Check sheet for the modelled part. Datum: model origin and axes. Units: mm. A direction names the side the tool comes from. Give positions to 0.01 mm unless a question says otherwise; leave off trailing zeros. Loops run counter-clockwise (first coordinate to the right, second up) from the corner with the lowest first, then second, coordinate; pieces in that order, holes last. Notation, with made-up numbers: (5, 5) - (33, 5) arc R4 cw to (33, 10) - close; hole circle Ø11 at (52.5, 16). An arc over 180 degrees is marked (long way). Answer in a Markdown table with one row per item. Add a question column.
(1) Sectioned sample at D-D on z = 4.75. Enter the section's corners in (x, y), then the cut area to 3 significant figures.
(2) Sectioned sample at B-B on z = 8.75. Enter the section's corners in (x, y).
(3) Sectioned sample at C-C on x = -11. Enter the section's corners in (y, z), then the cut area to 3 significant figures.
(4) Draft check along X on faces 5 (the face through (-19.3, -2, 1)), 6 (the face through (-20, 16, 0)), 7 (the face through (-22.3, -7, 3)), 8 (the face through (22.3, -7, 3)). Enter one of: released by +X, released by -X, zero draft, split by the parting line, or undercut.
(5) Set-up check for faces 1 (the face through (-13, -3, 2)), 2 (the face through (19.3, -2, 1)), 3 (the face through (-20, 0, 3.8)), 4 (the face through (11.5, -1, 9)): record each of +Z, -Z, +X, -X, +Y, -Y from which the full face is reachable in a straight line by a thin tool's end or side.
(6) Thickness scan on L1, parallel to X at y = 4, z = 2.75; L2, parallel to Z at x = -18, y = -15; L3, parallel to X at y = -3, z = 8.25. Record the ranges inside material, lowest first.
(7) Sectioned sample at A-A on y = 12. Enter the section's corners in (x, z), then the cut area to 3 significant figures.
(8) Go/stop test with flat-tipped pins: P1, Ø4, axis at x = -20, y = -2.5, coming from the +Z side; P2, Ø3, axis at y = -4, z = 7.5, coming from the -X side. Record where each tip stops, or that it passes through.
from build123d import *

# Parameters (mm, degrees)
BOSS_EXTRUDE1_DEPTH   = 35
BOSS_EXTRUDE1_2_DEPTH = 35
SKETCH1_W             = 2.5
SKETCH1_H             = 14
BOSS_EXTRUDE1_3_DEPTH = 35
BOSS_EXTRUDE1_4_DEPTH = 35
SKETCH2_W             = 44.6
SKETCH2_H             = 18.8
BOSS_EXTRUDE2_DEPTH   = 2.5
FILLET1_R             = 2
FILLET2_R             = 4


with BuildPart() as part:
    # Sketch1 → Boss-Extrude1 (new body)
    with BuildSketch(Plane(origin=(0, -19, 0), x_dir=(1, 0, 0), z_dir=(0, 1, 0))):
        Polygon((-19.3, 0.3), (-17.3, 0.3), (-17.3, 2.8), (-22.3, 2.8), (-22.3, -3.8), (-17.3, -3.8), (-17.3, -1.3), (-19.3, -1.3), align=None)
    extrude(amount=BOSS_EXTRUDE1_DEPTH)



with BuildPart() as body_2:
    # Sketch1 → Boss-Extrude1 2 (new body)
    with BuildSketch(Plane(origin=(0, -19, 0), x_dir=(1, 0, 0), z_dir=(0, 1, 0))):
        Polygon((19.3, -1.3), (19.3, 0.3), (17.3, 0.3), (17.3, 2.8), (22.3, 2.8), (22.3, -3.8), (17.3, -3.8), (17.3, -1.3), align=None)
    extrude(amount=BOSS_EXTRUDE1_2_DEPTH)


with BuildPart() as body_3:
    # Sketch1 → Boss-Extrude1 3 (new body)
    with BuildSketch(Plane(origin=(0, -19, 0), x_dir=(1, 0, 0), z_dir=(0, 1, 0))):
        with Locations((12.75, -9)):
            Rectangle(SKETCH1_W, SKETCH1_H)
    extrude(amount=BOSS_EXTRUDE1_3_DEPTH)


with BuildPart() as body_4:
    # Sketch1 → Boss-Extrude1 4 (new body)
    with BuildSketch(Plane(origin=(0, -19, 0), x_dir=(1, 0, 0), z_dir=(0, 1, 0))):
        with Locations((-12.75, -9)):
            Rectangle(SKETCH1_W, SKETCH1_H)
    extrude(amount=BOSS_EXTRUDE1_4_DEPTH)


with BuildPart() as part_1:
    add(part.part)

    add(body_2.part)  # Boss-Extrude2 merges body 2

    add(body_3.part)  # Boss-Extrude2 merges body 3

    add(body_4.part)  # Boss-Extrude2 merges body 4
    # Sketch2 → Boss-Extrude2 (add)
    with BuildSketch(Plane(origin=(0, -19, 0), x_dir=(1, 0, 0), z_dir=(0, 1, 0))):
        with Locations((0, -6.6)):
            Rectangle(SKETCH2_W, SKETCH2_H)
    extrude(amount=-BOSS_EXTRUDE2_DEPTH)

    # Fillet1
    fillet1_edges = [part_1.edges().sort_by_distance(p)[0] for p in [
        (11.5, -19, 9),
        (14, -19, 9),
        (-14, -19, 9),
        (-11.5, -19, 9),
    ]]
    fillet(fillet1_edges, radius=FILLET1_R)

    # Fillet2
    fillet2_edges = [part_1.edges().sort_by_distance(p)[0] for p in [
        (19.8, -19, 3.8),
        (-19.8, -19, 3.8),
    ]]
    fillet(fillet2_edges, radius=FILLET2_R)


solid = part_1.part
Reply:
| question | item | result |
|---|---|---|
| 1 | outline | (-22.3, -21.5) - (22.3, -21.5) - (22.3, -17.59) - (17.3, -17.59) - (17.3, -19) - (16, -19) arc R2 cw to (14, -17) - (14, 16) - (11.5, 16) - (11.5, -17) arc R2 cw to (9.5, -19) - (-9.5, -19) arc R2 cw to (-11.5, -17) - (-11.5, 16) - (-14, 16) - (-14, -17) arc R2 cw to (-16, -19) - (-17.3, -19) - (-17.3, -17.59) - (-22.3, -17.59) - close |
| 1 | area | 304 mm^2 |
| 2 | outline | (-22.3, -21.5) - (22.3, -21.5) - (22.3, -19) - (16, -19) arc R2 cw to (14, -17) - (14, 16) - (11.5, 16) - (11.5, -17) arc R2 cw to (9.5, -19) - (-9.5, -19) arc R2 cw to (-11.5, -17) - (-11.5, 16) - (-14, 16) - (-14, -17) arc R2 cw to (-16, -19) - (-22.3, -19) - close |
| 3 | outline | (-21.5, -2.8) - (-19, -2.8) - (-19, 2) - (-18.32, 2) - (-18.32, 16) - (-21.5, 16) - close |
| 3 | area | 56.5 mm^2 |
| 4 | face 5 | undercut |
| 4 | face 6 | zero draft |
| 4 | face 7 | released by -X |
| 4 | face 8 | released by +X |
| 5 | face 1 | -Z, +Y |
| 5 | face 2 | +Y |
| 5 | face 3 | +Z, -X, +Y |
| 5 | face 4 | +Z, -Z, +Y |
| 6 | L1 | -22.3 to -17.3, -14 to -11.5, 11.5 to 14, 17.3 to 22.3 |
| 6 | L2 | -2.8 to -0.3, 1.3 to 3.8 |
| 6 | L3 | -14 to -11.5, 11.5 to 14 |
| 7 | outline | (-22.3, -2.8) - (-17.3, -2.8) - (-17.3, -0.3) - (-19.3, -0.3) - (-19.3, 1.3) - (-17.3, 1.3) - (-17.3, 3.8) - (-22.3, 3.8) - close; (-14, 2) - (-11.5, 2) - (-11.5, 16) - (-14, 16) - close; (11.5, 2) - (14, 2) - (14, 16) - (11.5, 16) - close; (17.3, -2.8) - (22.3, -2.8) - (22.3, 3.8) - (17.3, 3.8) - (17.3, 1.3) - (19.3, 1.3) - (19.3, -0.3) - (17.3, -0.3) - close |
| 7 | area | 130 mm^2 |
| 8 | P1 | z = 3.8 |
| 8 | P2 | x = -14 |
